```python
from build123d import *

# Parameters (mm, degrees)
SKETCH1_R           = 1.5
BOSS_EXTRUDE2_DEPTH = 3


with BuildPart() as part:
    # Sketch1 → Boss-Extrude2 (new body)
    with BuildSketch(Plane.XY):
        with BuildLine():
            Line((-70.814700779, 145.910525624), (-49.601497343, 167.12372906))
            ThreePointArc((-49.601497343, 167.12372906), (-46.065963437, 168.588195154), (-42.530429531, 167.12372906))
            add(Edge.make_bspline(
                [(-42.530429531, 167.12372906), (-18.276788233, 140.587500568), (55.757413054, 90.515729887), (129.791614341, 140.587500568), (154.045255639, 167.12372906)],
                knots=[0, 0, 0, 0, 0.5, 1, 1, 1, 1], degree=3))
            ThreePointArc((154.045255639, 167.12372906), (157.547403451, 168.588083689), (161.068794171, 167.170627808))
            Line((161.068794171, 167.170627808), (182.281997607, 145.957424373))
            ThreePointArc((182.281997607, 145.957424373), (183.793881516, 142.408377812), (182.329526886, 138.839457812))
            add(Edge.make_bspline(
                [(182.329526886, -57.736227358), (155.793298394, -33.48258606), (105.721527713, 40.551615227), (155.793298394, 114.585816515), (182.329526886, 138.839457812)],
                knots=[0, 0, 0, 0, 0.5, 1, 1, 1, 1], degree=3))
            ThreePointArc((182.329526886, -57.736227358), (183.79399298, -61.271761264), (182.329526886, -64.807295169))
            Line((182.329526886, -64.807295169), (161.116323451, -86.020498605))
            ThreePointArc((161.116323451, -86.020498605), (157.580789545, -87.484964699), (154.045255639, -86.020498605))
            add(Edge.make_bspline(
                [(-42.530429531, -86.020498605), (-18.276788233, -59.484270113), (55.757413054, -9.412499432), (129.791614341, -59.484270113), (154.045255639, -86.020498605)],
                knots=[0, 0, 0, 0, 0.5, 1, 1, 1, 1], degree=3))
            ThreePointArc((-42.530429531, -86.020498605), (-46.065963437, -87.484964699), (-49.601497343, -86.020498605))
            Line((-49.601497343, -86.020498605), (-70.814700779, -64.807295169))
            ThreePointArc((-70.814700779, -64.807295169), (-72.279166873, -61.271761264), (-70.814700779, -57.736227358))
            add(Edge.make_bspline(
                [(-70.814700779, 138.839457812), (-44.278472287, 114.585816515), (5.793298394, 40.551615227), (-44.278472287, -33.48258606), (-70.814700779, -57.736227358)],
                knots=[0, 0, 0, 0, 0.5, 1, 1, 1, 1], degree=3))
            ThreePointArc((-70.814700779, 138.839457812), (-72.279166873, 142.374991718), (-70.814700779, 145.910525624))
        make_face()
        with Locations((-12.242586946, 40.551615227)):
            Circle(SKETCH1_R, mode=Mode.SUBTRACT)
        with Locations((55.757413054, 108.551615227)):
            Circle(SKETCH1_R, mode=Mode.SUBTRACT)
        with Locations((123.757413054, 40.551615227)):
            Circle(SKETCH1_R, mode=Mode.SUBTRACT)
        with Locations((55.757413054, -27.448384773)):
            Circle(SKETCH1_R, mode=Mode.SUBTRACT)
        with Locations((131.632800586, 75.501362696)):
            Circle(SKETCH1_R, mode=Mode.SUBTRACT)
        with Locations((131.632800586, 5.601867759)):
            Circle(SKETCH1_R, mode=Mode.SUBTRACT)
        with Locations((20.807665586, 116.427002759)):
            Circle(SKETCH1_R, mode=Mode.SUBTRACT)
        with Locations((90.707160522, 116.427002759)):
            Circle(SKETCH1_R, mode=Mode.SUBTRACT)
        with Locations((-20.117974478, 75.501362696)):
            Circle(SKETCH1_R, mode=Mode.SUBTRACT)
        with Locations((-20.117974478, 5.601867759)):
            Circle(SKETCH1_R, mode=Mode.SUBTRACT)
        with Locations((20.807665586, -35.323772305)):
            Circle(SKETCH1_R, mode=Mode.SUBTRACT)
        with Locations((90.707160522, -35.323772305)):
            Circle(SKETCH1_R, mode=Mode.SUBTRACT)
        with Locations((-67.279166873, 142.374991718)):
            Circle(SKETCH1_R, mode=Mode.SUBTRACT)
        with Locations((-46.065963437, 163.588195154)):
            Circle(SKETCH1_R, mode=Mode.SUBTRACT)
        with Locations((157.580789545, 163.588195154)):
            Circle(SKETCH1_R, mode=Mode.SUBTRACT)
        with Locations((157.580789545, -82.484964699)):
            Circle(SKETCH1_R, mode=Mode.SUBTRACT)
        with Locations((178.79399298, -61.271761264)):
            Circle(SKETCH1_R, mode=Mode.SUBTRACT)
        with Locations((-67.279166873, -61.271761264)):
            Circle(SKETCH1_R, mode=Mode.SUBTRACT)
        with Locations((-46.065963437, -82.484964699)):
            Circle(SKETCH1_R, mode=Mode.SUBTRACT)
        with Locations((178.79399298, 142.374991718)):
            Circle(SKETCH1_R, mode=Mode.SUBTRACT)
        with Locations((-53.137031249, 128.232856094)):
            Circle(SKETCH1_R, mode=Mode.SUBTRACT)
        with Locations((-31.923827813, 149.44605953)):
            Circle(SKETCH1_R, mode=Mode.SUBTRACT)
        with Locations((143.438653921, 149.44605953)):
            Circle(SKETCH1_R, mode=Mode.SUBTRACT)
        with Locations((164.651857357, 128.232856094)):
            Circle(SKETCH1_R, mode=Mode.SUBTRACT)
        with Locations((143.438653921, -68.342829075)):
            Circle(SKETCH1_R, mode=Mode.SUBTRACT)
        with Locations((164.651857357, -47.12962564)):
            Circle(SKETCH1_R, mode=Mode.SUBTRACT)
        with Locations((-53.137031249, -47.12962564)):
            Circle(SKETCH1_R, mode=Mode.SUBTRACT)
        with Locations((-31.923827813, -68.342829075)):
            Circle(SKETCH1_R, mode=Mode.SUBTRACT)
    extrude(amount=BOSS_EXTRUDE2_DEPTH)


solid = part.part
```
Can you work these out from the model? Positions are in its coordinate system, mm. Coordinates: 2 decimals unless noted, no trailing zeros. Put each result on its own line as item: value. Start each with the question number.
Q1. I want a section at A-A (z = 1.7). Count the separate pieces of the cut face and the enclosed holes in it, plus the area to 3 significant figures.
Q2. If I drill on line 1 (X direction, y = 75, z = 1.8); line 2 (Y direction, x = 91, z = 2.55); line 3 (Y direction, x = 90, z = 1), over which ranges is the centre line in solid material (lowest first)? Write a range as [from, to].
Q3. I'm going to push flat-ended pins straight in: P1, Ø4, axis at x = -31.92, y = -68.34, coming from the +Z side; P2, Ø1.5, axis at x = 127, z = 1, coming from the +Y side; P3, Ø1.5, axis at y = 125.5, z = 1, coming from the -X side; P4, Ø1.5, axis at x = 19, z = 2.5, coming from the +Y side. Where does each tip first touch, or does it pass through?
Taken from the geometry:
1. separate pieces: 1
1. enclosed holes: 28
1. area: 36,100 mm2
2. line 1: x = [-25.91, -21.53], [-18.7, 130.22], [133.05, 137.42]
2. line 2: y = [-41.42, -36.79], [-33.85, 114.96], [117.9, 122.52]
2. line 3: y = [-41.04, -36.65], [-34, 115.1], [117.75, 122.14]
3. P1: stops at z = 3
3. P2: stops at y = 143.25
3. P3: stops at x = -58.27
3. P4: stops at y = 123.41
